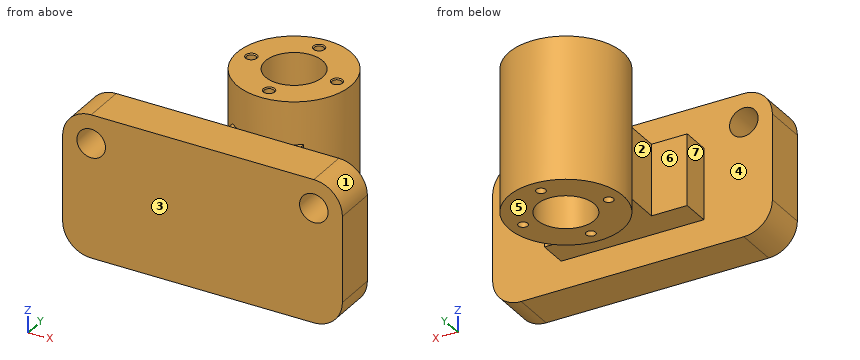
```python
from build123d import *

# Parameters (mm, degrees)
SKETCH_1_W                   = 98
SKETCH_1_H                   = 15
EXTRUDE_1_DEPTH              = 50
SKETCH_2_R                   = 20
SKETCH_2_R_2                 = 10
EXTRUDE_2_DEPTH              = 50
SKETCH_4_W                   = 25
SKETCH_4_H                   = 24.3455958
EXTRUDE_3_DEPTH              = 12.5
FILLET_1_R                   = 10
SKETCH_7_R                   = 5
CUT_EXTRUDE_1_DEPTH          = 25
HOLE_WIZARD_M4_1_D           = 3.3
HOLE_WIZARD_M4_1_CSINK_D     = 4.05
HOLE_WIZARD_M4_1_CSINK_ANGLE = 92
SKETCH_12_W                  = 50
SKETCH_12_H                  = 10
EXTRUDE_4_DEPTH              = 25


with BuildPart() as part:
    # Sketch 1 → Extrude 1 (new body)
    with BuildSketch(Plane.XY):
        with Locations((0, -27.507396928)):
            Rectangle(SKETCH_1_W, SKETCH_1_H)
    extrude(amount=EXTRUDE_1_DEPTH)



with BuildPart() as body_2:
    # Sketch 2 → Extrude 2 (new body)
    with BuildSketch(Plane.XY.offset(50)):
        with Locations((0, 19.992603072)):
            Circle(SKETCH_2_R)
        with Locations((0, 19.992603072)):
            Circle(SKETCH_2_R_2, mode=Mode.SUBTRACT)
    extrude(amount=-EXTRUDE_2_DEPTH)


with BuildPart() as part_1:
    add(part.part)

    add(body_2.part)  # Extrude 3 merges body 2
    # Sketch 4 → Extrude 3 (add, symmetric)
    with BuildSketch(Plane(origin=(0, 0, 0), x_dir=(0, 0, -1), z_dir=(1, 0, 0))):
        with Locations((-22.5, -7.834599028)):
            Rectangle(SKETCH_4_W, SKETCH_4_H)
    extrude(amount=EXTRUDE_3_DEPTH, both=True)

    # Fillet 1
    fillet_1_edges = [part_1.edges().sort_by_distance(p)[0] for p in [
        (-49, -27.507396928, 50),
        (49, -27.507396928, 50),
        (-49, -27.507396928, 0),
        (49, -27.507396928, 0),
    ]]
    fillet(fillet_1_edges, radius=FILLET_1_R)

    # Sketch 7 → Cut-Extrude 1 (cut)
    with BuildSketch(Plane(origin=(0, -20.007396928, 0), x_dir=(1, 0, 0), z_dir=(0, 1, 0))):
        with Locations(Location((-39, -40, 0), (0, 0, 270))):
            Circle(SKETCH_7_R)
        with Locations(Location((39, -40, 0), (0, 0, 270))):
            Circle(SKETCH_7_R)
    extrude(amount=-CUT_EXTRUDE_1_DEPTH, mode=Mode.SUBTRACT)

    # Hole Wizard M4 _ _1 (through all)
    with Locations(Plane(origin=(0, 34.992603072, 50), x_dir=(1, 0, 0), z_dir=(0, 0, 1))):
        with Locations((0, 0), (-15, -15), (15, -15), (0, -30)):
            CounterSinkHole(HOLE_WIZARD_M4_1_D / 2, HOLE_WIZARD_M4_1_CSINK_D / 2, counter_sink_angle=HOLE_WIZARD_M4_1_CSINK_ANGLE)

    # Sketch 12 → Extrude 4 (add)
    with BuildSketch(Plane.XY.offset(35)):
        with Locations((0, -15.007396928)):
            Rectangle(SKETCH_12_W, SKETCH_12_H)
    extrude(amount=-EXTRUDE_4_DEPTH)


solid = part_1.part
```
Part model, mm, in its own coordinate system. Face numbers are marked on the shaded views. A direction names the side the tool comes from. Round coordinates to 2 decimals unless told otherwise and drop trailing zeros. Loops run counter-clockwise (first coordinate to the right, second up) from the corner with the lowest first, then second, coordinate; pieces in that order, holes last. Notation, with made-up numbers: (-9.75, -33) -> (6.25, -33) arc R20 ccw to (6.25, -8) -> close; hole circle Ø6 at (44.25, -2). An arc over 180 degrees is marked (long way). Use a Markdown table: item, result.
1) Cut at D-D, the plane x = -15. List the corners of the cut face in (y, z).
The answers:
| item | result |
|---|---|
| outline | (-35.01, 0) -> (-20.01, 0) -> (-20.01, 10) -> (-10.01, 10) -> (-10.01, 35) -> (-20.01, 35) -> (-20.01, 50) -> (-35.01, 50) -> close; (6.76, 0) -> (18.34, 0) -> (18.34, 49.64) -> (17.97, 50) -> (6.76, 50) -> close; (21.64, 0) -> (33.22, 0) -> (33.22, 50) -> (22.02, 50) -> (21.64, 49.64) -> close |
2) Cut at C-C, the plane z = 8.5. List the corners of the cut face in (x, y), and give its area (3 significant figures).
The answers:
| item | result |
|---|---|
| outline | (-48.89, -35.01) -> (48.89, -35.01) -> (48.89, -20.01) -> (-48.89, -20.01) -> close; circle Ø40 at (0, 19.99); hole circle Ø3.3 at (-15, 19.99); hole circle Ø20 at (0, 19.99); hole circle Ø3.3 at (0, 4.99); hole circle Ø3.3 at (0, 34.99); hole circle Ø3.3 at (15, 19.99) |
| area | 2,370 mm2 |
3) Pull direction Y, two halves, no side cores. Call the marked faces 1, 2, 3 and 4: pulls with the +Y half, pulls with the -Y half, needs draft (parallel to the pull), parting line crosses it, or undercut.
The answers:
| item | result |
|---|---|
| face 1 | needs draft |
| face 2 | undercut |
| face 3 | pulls with the -Y half |
| face 4 | undercut |
4) Drop flat-ended pins along their axis: pin 1 Ø6 at (x, z) = (-39, 40) entering from -Y; pin 2 Ø4.5 at (y, z) = (-3, 28) entering from +X; pin 3 Ø6 at (x, z) = (-18.5, 21) entering from +Y; pin 4 Ø5 at (y, z) = (-13.5, 24) entering from -X. Give the stop position or say it passes through.
The answers:
| item | result |
|---|---|
| pin 1 | passes through |
| pin 2 | stops at x = 12.5 |
| pin 3 | stops at y = 32.63 |
| pin 4 | stops at x = -25 |
5) Cut at A-A, the plane y = -27. List the corners of the cut face in (x, z), and give its area (3 significant figures).
The answers:
| item | result |
|---|---|
| outline | (-49, 10) arc R10 ccw to (-39, 0) -> (39, 0) arc R10 ccw to (49, 10) -> (49, 40) arc R10 ccw to (39, 50) -> (-39, 50) arc R10 ccw to (-49, 40) -> close; hole circle Ø10 at (-39, 40); hole circle Ø10 at (39, 40) |
| area | 4,660 mm2 |
6) Tool access for the marked faces 5, 6 and 7: list every direction of +Z, -Z, +X, -X, +Y, -Y with a clear straight run to the whole face (end or side of a thin tool).
The answers:
| item | result |
|---|---|
| face 5 | -Z, +X, -X, +Y, -Y |
| face 6 | +Z, -Z, -X |
| face 7 | +Z, -Z, -X, +Y |
7) Probe line 1 (X direction, y = -26.25, z = 40); line 2 (Y direction, x = 0, z = 34); line 3 (X direction, y = 20, z = 33). List the from-to ranges inside material, lowest first. Write a range as [from, to].
The answers:
| item | result |
|---|---|
| line 1 | x = [-49, -44], [-34, 34], [44, 49] |
| line 2 | y = [-35.01, 3.34], [6.64, 9.99], [29.99, 33.34], [36.64, 39.99] |
| line 3 | x = [-20, -16.65], [-13.35, -10], [10, 13.35], [16.65, 20] |
8) Cut at B-B, the plane x = 0. List the corners of the cut face in (y, z), and give its area (3 significant figures).
The answers:
| item | result |
|---|---|
| outline | (-35.01, 0) -> (-20.01, 0) -> (-20.01, 10) -> (-0.01, 10) -> (-0.01, 0) -> (3.34, 0) -> (3.34, 49.64) -> (2.97, 50) -> (-0.01, 50) -> (-0.01, 35) -> (-20.01, 35) -> (-20.01, 50) -> (-35.01, 50) -> close; (6.64, 0) -> (9.99, 0) -> (9.99, 50) -> (7.02, 50) -> (6.64, 49.64) -> close; (29.99, 0) -> (33.34, 0) -> (33.34, 49.64) -> (32.97, 50) -> (29.99, 50) -> close; (36.64, 0) -> (39.99, 0) -> (39.99, 50) -> (37.02, 50) -> (36.64, 49.64) -> close |
| area | 1,920 mm2 |
